The model under review builds one solid part; all positions refer to its coordinate system, in mm. Face numbers are marked on the shaded views. A direction names the side the tool comes from. Coordinates: 2 decimals unless noted, no trailing zeros. Order: outer loops, then holes, each group sorted by start corner. A loop starts at its lowest first (then second) coordinate and runs counter-clockwise, first axis right, second up. Notation, with made-up numbers: (-15.5, -30) - (41.5, -30) arc R34 ccw to (41.5, 9) - close; hole circle Ø11 at (16.25, -18.5). An arc over 180 degrees is marked (long way). Answer in a Markdown table with one row per item.
```python
from build123d import *

# Parameters (mm, degrees)
SKETCH1_W           = 10
SKETCH1_H           = 10
SKETCH1_R           = 1.25
BOSS_EXTRUDE1_DEPTH = 1
SKETCH2_R           = 4
SKETCH2_R_2         = 1.51
BOSS_EXTRUDE2_DEPTH = 8.525


with BuildPart() as part:
    # Sketch1 → Boss-Extrude1 (new body)
    with BuildSketch(Plane(origin=(0, 0, 0), x_dir=(1, 0, 0), z_dir=(0, 1, 0))):
        with Locations((5, -5)):
            Rectangle(SKETCH1_W, SKETCH1_H)
        with Locations((5, -5)):
            Circle(SKETCH1_R, mode=Mode.SUBTRACT)
    extrude(amount=BOSS_EXTRUDE1_DEPTH)

    # Sketch2 → Boss-Extrude2 (add)
    with BuildSketch(Plane(origin=(0, 1, 0), x_dir=(1, 0, 0), z_dir=(0, 1, 0))):
        with Locations((5, -5)):
            Circle(SKETCH2_R)
        with Locations((5, -5)):
            Circle(SKETCH2_R_2, mode=Mode.SUBTRACT)
    extrude(amount=BOSS_EXTRUDE2_DEPTH)


solid = part.part
```
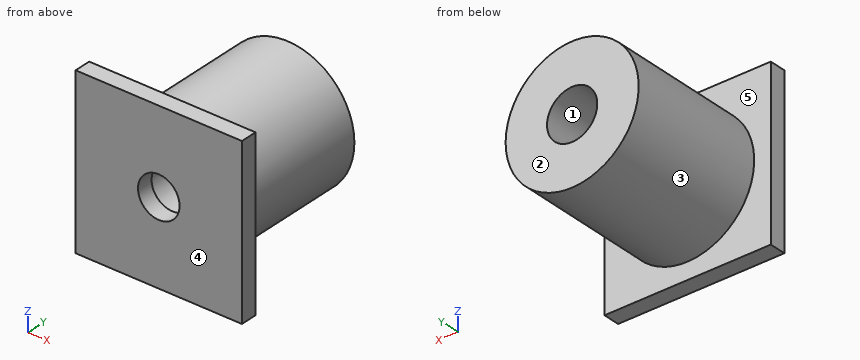
Item 1: Tool access review of the marked faces 4 and 5: name each direction out of +Z, -Z, +X, -X, +Y, -Y from which nothing blocks a thin tool from reaching the whole face with its end or side.
Check values:
| item | result |
|---|---|
| face 4 | +Z, -Z, +X, -X, -Y |
| face 5 | +Y |
Item 2: Mouldability with a two-part tool opening along X and no side actions: class the marked faces 1, 2 and 3 as +X half, -X half, draft (parallel to the pull), parting line (faces both ways), or undercut.
Check values:
| item | result |
|---|---|
| face 1 | undercut |
| face 2 | draft |
| face 3 | parting line |
Item 3: We need section D-D, the plane z = 7.25. Write out the cut boundary in (x, y) (3 decimals).
Check values:
| item | result |
|---|---|
| outline | (0, 0) - (10, 0) - (10, 1) - (8.307, 1) - (8.307, 9.525) - (1.693, 9.525) - (1.693, 1) - (0, 1) - close |
Item 4: We need section C-C, the plane y = 8. Write out the cut boundary in (x, z), then the cut area to 3 significant figures.
Check values:
| item | result |
|---|---|
| outline | circle Ø8 at (5, 5); hole circle Ø3.02 at (5, 5) |
| area | 43.1 mm^2 |
Item 5: To check wall thickness, follow line 1 (Z direction, x = 5, y = 3.25); line 2 (X direction, y = 0.8, z = 5). State the ranges of each line that lie inside material, in increasing order. Write a range as from..to.
Check values:
| item | result |
|---|---|
| line 1 | 1..3.49, 6.51..9 |
| line 2 | 0..3.75, 6.25..10 |
Item 6: We need section B-B, the plane z = 5. Write out the cut boundary in (x, y) (3 decimals).
Check values:
| item | result |
|---|---|
| outline | (0, 0) - (3.75, 0) - (3.75, 1) - (3.49, 1) - (3.49, 9.525) - (1, 9.525) - (1, 1) - (0, 1) - close; (6.25, 0) - (10, 0) - (10, 1) - (9, 1) - (9, 9.525) - (6.51, 9.525) - (6.51, 1) - (6.25, 1) - close |
Item 7: Clearance check with flat-ended pins moving along their axes: pin 1 Ø1.5 at (x, y) = (4.5, 4.5) entering from -Z; pin 2 Ø1 at (y, z) = (3.5, 5) entering from +X; pin 3 Ø2 at (x, z) = (3, 3) entering from -Y; pin 4 Ø4 at (x, y) = (8.5, 5) entering from -Z. State where each tip first meets the part, or that it passes through.
Check values:
| item | result |
|---|---|
| pin 1 | z = 1 |
| pin 2 | x = 9 |
| pin 3 | y = 0 |
| pin 4 | z = 1.29 |
Item 8: We need section A-A, the plane x = 5. Write out the cut boundary in (y, z) (3 decimals), then the cut area to 3 significant figures.
Check values:
| item | result |
|---|---|
| outline | (0, 0) - (1, 0) - (1, 1) - (9.525, 1) - (9.525, 3.49) - (1, 3.49) - (1, 3.75) - (0, 3.75) - close; (0, 6.25) - (1, 6.25) - (1, 6.51) - (9.525, 6.51) - (9.525, 9) - (1, 9) - (1, 10) - (0, 10) - close |
| area | 50.0 mm^2 |
